Can you work these out from the model? Positions are in its coordinate system, mm. Give positions to 0.01 mm unless a question says otherwise; leave off trailing zeros. Write each loop counter-clockwise with the first axis right and the second up, starting at its lowest first coordinate (ties: lowest second). Pieces come first, ordered by that corner, then holes. Notation, with made-up numbers: M 47,33.5 L 68,33.5 A28 ccw 68,57.5 Z; hole C 27,-15.75 d5. An arc over 180 degrees is marked long. Answer as CSV lines item,"result". Start each with the question number.
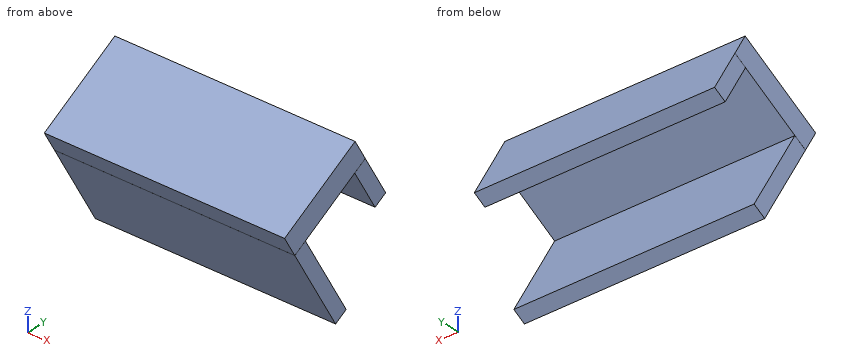
```python
from build123d import *

# Parameters (mm, degrees)
SKETCH057_W             = 50
SKETCH057_H             = 20
PAD056_DEPTH            = 5
SKETCH058_W             = 50
SKETCH058_H             = 3
PAD057_DEPTH            = 20
SKETCH059_W             = 50
SKETCH059_H             = 10
PAD058_DEPTH            = 3
BODY043_ROLL_ANGLE      = 149.965102
BODY043_PITCH_ANGLE     = -0.000568
BODY043_PLACEMENT_ANGLE = 179.999625


with BuildPart() as part:
    # Sketch057 → Pad056 (new body)
    with BuildSketch(Plane.XY):
        with Locations((184.845276, -123.914059)):
            Rectangle(SKETCH057_W, SKETCH057_H)
    extrude(amount=PAD056_DEPTH)

    # Sketch058 (on Face6 of Pad056) → Pad057 (join)
    with BuildSketch(Plane.XY.offset(5)):
        with Locations((184.83606, -132.417099)):
            Rectangle(SKETCH058_W, SKETCH058_H)
    extrude(amount=PAD057_DEPTH)

    # Sketch059 (on Face7 of Pad057) → Pad058 (join)
    with BuildSketch(Plane(origin=(0, -113.914059, 0), x_dir=(-1, 0, 0), z_dir=(0, 1, 0))):
        with Locations((-184.841869, 9.989668)):
            Rectangle(SKETCH059_W, SKETCH059_H)
    extrude(amount=-PAD058_DEPTH)


with BuildPart() as part_1:
    # Body043 roll: moved
    add(part.part.rotate(Axis((0, 0, 0), (1, 0, 0)), BODY043_ROLL_ANGLE))


with BuildPart() as part_2:
    # Body043 pitch: moved
    add(part_1.part.rotate(Axis((0, 0, 0), (0, 1, 0)), BODY043_PITCH_ANGLE))


with BuildPart() as part_3:
    # Body043 placement: moved
    add(part_2.part.moved(Location((186.038525, 90.64289, 266.847744))).rotate(Axis((186.038525, 90.64289, 266.847744), (0, 0, 1)), BODY043_PLACEMENT_ANGLE))


solid = part_3.part
```
1) I want a section at A-A, the plane z = 199. Please give me the cut outline in (x, y).
2) I want a section at B-B, the plane y = -17.5. Please give me the cut outline in (x, z), then the cut area to 3 significant figures.
3) I'm going to push flat-ended pins straight in: P1, Ø4, axis at y = -14, z = 204, coming from the +X side; P2, Ø1, axis at x = 14, z = 188.5, coming from the -Y side; P3, Ø12, axis at x = 6, z = 187, coming from the +Y side. Where does each tip first touch, or does it pass through?
4) I need wall thicknesses on L1, parallel to Y at x = 4.5, z = 200.5; L2, parallel to Y at x = -7.5, z = 196.5; L3, parallel to Z at x = -7, y = -19. Which ranges of each line are inside material? Lowest first, please. Write a range as from..to.
Values found:
1,outline,"M -23.81,-24.81 L 26.19,-24.81 L 26.19,-16.72 L -23.81,-16.72 Z; M -23.8,-5.18 L 26.2,-5.18 L 26.2,-1.71 L -23.8,-1.71 Z"
2,outline,"M -23.81,198.55 L 26.19,198.55 L 26.19,204.32 L -23.81,204.32 Z; M -23.8,186.35 L 26.2,186.34 L 26.2,192.34 L -23.8,192.34 Z"
2,area,"588 mm²"
3,P1,"stops at x = 26.19"
3,P2,"stops at y = -19.03"
3,P3,"stops at y = -10.94"
4,L1,"y = -24.12..-14.13, -6.04..-2.58"
4,L2,"y = -23.37..-19.91, -3.73..-1.09"
4,L3,"z = 188.94..194.93, 197.68..203.46"
